Design review of the part built by this model. Coordinates are the model's own, in mm. A direction names the side the tool comes from. Coordinates: 2 decimals unless noted, no trailing zeros. Order: outer loops, then holes, each group sorted by start corner. A loop starts at its lowest first (then second) coordinate and runs counter-clockwise, first axis right, second up. Notation, with made-up numbers: M 44,-32.75 L 65,-32.75 A20 cw 65,1.25 Z; hole C 11,35 d6. An arc over 180 degrees is marked long. Use CSV: the item, a comma, the result in double quotes.
```python
from build123d import *

# Parameters (mm, degrees)
SKETCH1_W                        = 39.9542
SKETCH1_H                        = 20.066
BOSS_EXTRUDE1_DEPTH              = 75.057
FILLET1_R                        = 1.016
F_1_4_20_TAPPED_HOLE1_AT_2_COUNT = 2
F_1_4_20_TAPPED_HOLE1_AT_2_PITCH = 19.685


with BuildPart() as part:
    # Sketch1 → Boss-Extrude1 (new, symmetric)
    with BuildSketch(Plane.XY):
        Rectangle(SKETCH1_W, SKETCH1_H)
    extrude(amount=BOSS_EXTRUDE1_DEPTH, both=True)

    # Fillet1
    fillet1_edges = [part.edges().sort_by_distance(p)[0] for p in [
        (19.9771, -10.033, 0),
        (-19.9771, -10.033, 0),
        (-19.9771, 10.033, 0),
        (19.9771, 10.033, 0),
    ]]
    fillet(fillet1_edges, radius=FILLET1_R)

    # Sketch4 → 1/4-20 Tapped Hole1 (revolve, cut)
    with BuildSketch(Plane(origin=(9.8425, 0, -75.057), x_dir=(0, 1, 0), z_dir=(1, 0, 0))):
        Polygon((0, 0), (0, 18.043816902), (2.5527, 16.51), (2.5527, 0), align=None)
    f_1_4_20_tapped_hole1 = revolve(axis=Axis((9.8425, 0, -81.407), (0, 0, 1)), mode=Mode.SUBTRACT)

    # 1/4-20 Tapped Hole1 at 2: 1/4-20 Tapped Hole1 ×2
    with Locations(*[(-i * F_1_4_20_TAPPED_HOLE1_AT_2_PITCH, 0, 0) for i in range(1, F_1_4_20_TAPPED_HOLE1_AT_2_COUNT)]):
        add(f_1_4_20_tapped_hole1, mode=Mode.SUBTRACT)

    # Mirror1: 1/4-20 Tapped Hole1 across plane
    add(f_1_4_20_tapped_hole1.mirror(Plane.XY), mode=Mode.SUBTRACT)

    # Mirror1 copy 1 sketch → Mirror1 copy 1 (revolve, cut)
    with BuildSketch(Plane(origin=(-9.8425, 0, 75.057), x_dir=(0, 1, 0), z_dir=(1, 0, 0))):
        Polygon((0, 0), (0, -18.043816902), (2.5527, -16.51), (2.5527, 0), align=None)
    revolve(axis=Axis((-9.8425, 0, 81.407), (0, 0, 1)), mode=Mode.SUBTRACT)


solid = part.part
```
(1) Clearance check with flat-ended pins moving along their axes: P1, Ø4.5, axis at x = -9.84, y = 0, coming from the -Z side; P2, Ø3, axis at x = 9.84, y = 0, coming from the -Z side. State where each tip first meets the part, or that it passes through.
The answers:
P1,"stops at z = -58.37"
P2,"stops at z = -57.92"
(2) The part is to be moulded in two halves that separate along X. For faces 4 (the face through (19.977, 0, 1)), 5 (the face through (-7.35, -0.55, 66.92)), 6 (the face through (0, 0, 75.057)), say which applies: pulls with the +X half, pulls with the -X half, needs draft (parallel to the pull), parting line crosses it, or undercut.
The answers:
face 4,"pulls with the +X half"
face 5,"undercut"
face 6,"needs draft"
(3) Wall thickness on probe 1 along X at (y, z) = (0.25, -64); probe 2 along Y at (x, z) = (-12, -64.5); probe 3 along Z at (x, y) = (10.5, 1.5): over which ranges is each line inside the solid? List them lowest first.
The answers:
probe 1,"x = -19.98 to -12.38, -7.3 to 7.3, 12.38 to 19.98"
probe 2,"y = -10.03 to -1.36, 1.36 to 10.03"
probe 3,"z = -58 to 58"
(4) For faces 1 (the face through (0, 0, -75.057)), 2 (the face through (7.31, -0.33, 66.92)), 3 (the face through (-7.58, 1.18, -66.92)), list the 3-axis set-ups (+Z, -Z, +X, -X, +Y, -Y) from which the entire face can be reached by the end or side of a thin tool; tool diameter is ignored.
The answers:
face 1,"-Z, +X, -X, +Y, -Y"
face 2,"+Z"
face 3,"-Z"
(5) Add section A-A on z = 61. State the section outline as (x, y) points, and give its area (3 significant figures).
The answers:
outline,"M -19.98,-9.02 A1.02 ccw -18.96,-10.03 L 18.96,-10.03 A1.02 ccw 19.98,-9.02 L 19.98,9.02 A1.02 ccw 18.96,10.03 L -18.96,10.03 A1.02 ccw -19.98,9.02 Z; hole C -9.84,0 d5.11; hole C 9.84,0 d5.11"
area,"760 mm2"
